Could you check a few things on this model? Use its own coordinates, in mm. A direction names the side the tool comes from. Coordinates: 2 decimals unless noted, no trailing zeros. Write each loop counter-clockwise with the first axis right and the second up, starting at its lowest first coordinate (ties: lowest second). Pieces come first, ordered by that corner, then holes.
```python
from build123d import *

# Parameters (mm, degrees)
F0_R     = 17
F1_DEPTH = 8
F2_R     = 15
F3_DEPTH = 8
F4_R     = 17
F5_DEPTH = 1
F6_R     = 13
F7_DEPTH = 1
F8_R     = 0.99999
F9_R     = 1


# Not quite as in the source:
# - a fillet or chamfer is up to 0.001 mm smaller than in the source, because OpenCascade refuses the exact size


with BuildPart() as f1:
    # F0 (on Top) → F1 (new body)
    with BuildSketch(Plane.XY):
        Circle(F0_R)
    extrude(amount=F1_DEPTH)

    # F2 (on face) → F3 (cut)
    with BuildSketch(Plane(origin=(0, 0, 0), x_dir=(1, 0, 0), z_dir=(0, 0, -1))):
        Circle(F2_R)
    extrude(amount=-F3_DEPTH, mode=Mode.SUBTRACT)

    # F4 (on face) → F5 (join)
    with BuildSketch(Plane.XY.offset(8)):
        Circle(F4_R)
    extrude(amount=F5_DEPTH)

    # F6 (on face) → F7 (cut)
    with BuildSketch(Plane.XY.offset(9)):
        Circle(F6_R)
    extrude(amount=-F7_DEPTH, mode=Mode.SUBTRACT)

    # F8 (radius 1 in the source; OpenCascade refuses exactly that, so slightly less here)
    f8_edges = [f1.edges().sort_by_distance(p)[0] for p in [
        (-17, 0, 0),
        (-15, 0, 0),
    ]]
    fillet(f8_edges, radius=F8_R)

    # F9
    f9_edges = [f1.edges().sort_by_distance(p)[0] for p in [
        (-17, 0, 9),
    ]]
    fillet(f9_edges, radius=F9_R)


solid = f1.part
```
1. I want a section at C-C on z = 6.5. Please give me the cut outline in (x, y), plus the area to 3 significant figures.
Verdict:
outline: circle Ø34 at (0, 0); hole circle Ø30 at (0, 0)
area: 201 mm2
2. Please list where these lines run through material, in increasing order: line 1 along Y through (x, z) = (0, 3.25); line 2 along Y through (x, z) = (-9, 4.5); line 3 along Z through (x, y) = (-12, 6).
Verdict:
line 1: y = -17 to -15, 15 to 17
line 2: y = -14.42 to -12, 12 to 14.42
line 3: z = 8 to 9
3. On a 3-axis mill with a long thin cutter (end or side, diameter ignored), from which of +Z, -Z, +X, -X, +Y, -Y can I reach the whole of each face in a straight line? I mean faces 1 (the face through (-10.316, -7.91, 8.507)), 2 (the face through (-14.985, -0.66, 4.451)). Say none if no direction works.
Verdict:
face 1: +Z, -Z
face 2: -Z
4. If we mould it in two halves opening along Y, with no side actions, what happens to faces 3 (the face through (9.139, 14.334, 4.451)), 4 (the face through (-1.3, 13.1, 9)), 5 (the face through (-0.1, 13.4, 8))? For each: pulls with the +Y half, pulls with the -Y half, needs draft (parallel to the pull), parting line crosses it, or undercut.
Verdict:
face 3: parting line crosses it
face 4: needs draft
face 5: undercut
5. For pin 1 (3 mm diameter, centred on y = 5, z = 3.5, fed in from -X); pin 2 (1.5 mm diameter, centred on x = 13.5, y = -9, fed in from -Z); pin 3 (5 mm diameter, centred on y = -9, z = 7.5, fed in from -X); pin 4 (2 mm diameter, centred on x = -8, z = 1.5, fed in from +Y), each with a flat end and sliding along its axis, tell me the tip position at first contact or that it passes through.
Verdict:
pin 1: stops at x = -16.64
pin 2: stops at z = 0
pin 3: stops at x = -15.71
pin 4: stops at y = 15.49
